Design review of the part built by this model. Coordinates are the model's own, in mm. Face numbers are marked on the shaded views. Give positions to 0.01 mm unless a question says otherwise; leave off trailing zeros. Order: outer loops, then holes, each group sorted by start corner. A loop starts at its lowest first (then second) coordinate and runs counter-clockwise, first axis right, second up. Notation, with made-up numbers: (18, -31) -> (59, -31) arc R11 cw to (59, -16) -> close; hole circle Ø10 at (40.5, -26.5). An arc over 180 degrees is marked (long way). Return JSON: item names as keys, results as strings.
```python
from build123d import *

# Parameters (mm, degrees)
SKETCH1_R           = 35.814
SKETCH1_R_2         = 2.032
BOSS_EXTRUDE1_DEPTH = 50.292
SKETCH2_R           = 13.716
CUT_EXTRUDE1_DEPTH  = 31.75
FILLET1_R           = 2.032


with BuildPart() as part:
    # Sketch1 → Boss-Extrude1 (new body)
    with BuildSketch(Plane(origin=(0, 0, 0), x_dir=(1, 0, 0), z_dir=(0, 1, 0))):
        with Locations(Location((0, 0, 0), (0, 0, 270))):
            Circle(SKETCH1_R)
        with Locations(Location((-20.308177359, -15.255750796, 0), (0, 0, 270))):
            Circle(SKETCH1_R_2, mode=Mode.SUBTRACT)
        with Locations(Location((-3.057779064, 25.215272896, 0), (0, 0, 270))):
            Circle(SKETCH1_R_2, mode=Mode.SUBTRACT)
        with Locations(Location((23.365956423, -9.959522099, 0), (0, 0, 270))):
            Circle(SKETCH1_R_2, mode=Mode.SUBTRACT)
    extrude(amount=BOSS_EXTRUDE1_DEPTH)

    # Sketch2 → Cut-Extrude1 (cut)
    with BuildSketch(Plane(origin=(0, 50.292, 0), x_dir=(1, 0, 0), z_dir=(0, 1, 0))):
        with Locations(Location((0, 0, 0), (0, 0, 270))):
            Circle(SKETCH2_R)
    extrude(amount=-CUT_EXTRUDE1_DEPTH, mode=Mode.SUBTRACT)

    # Fillet1
    fillet1_edges = [part.edges().sort_by_distance(p)[0] for p in [
        (0, 50.292, -35.814),
    ]]
    fillet(fillet1_edges, radius=FILLET1_R)


solid = part.part
```
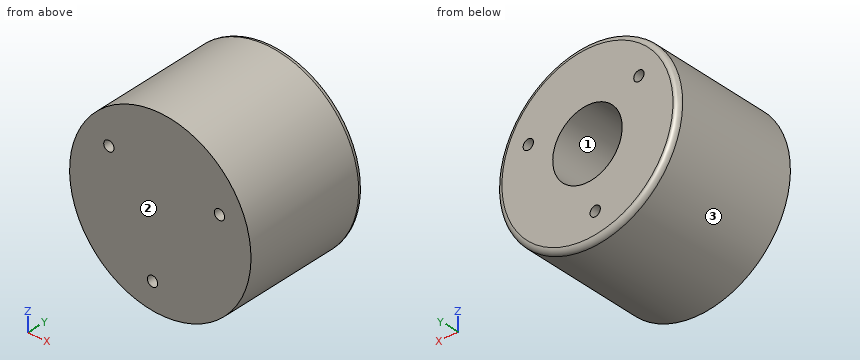
Item 1: Add section A-A (z = 0). Give the boundary of the cut face in (x, y).
Result set:
{"outline": "(-35.81, 0) -> (35.81, 0) -> (35.81, 48.26) arc R2.03 ccw to (33.78, 50.29) -> (13.72, 50.29) -> (13.72, 18.54) -> (-13.72, 18.54) -> (-13.72, 50.29) -> (-33.78, 50.29) arc R2.03 ccw to (-35.81, 48.26) -> close"}
Item 2: For pin 1 (8 mm diameter, centred on x = -4.5, y = 7.5, fed in from +Z); pin 2 (1 mm diameter, centred on x = -14.5, y = 14, fed in from -Z); pin 3 (5 mm diameter, centred on x = 23, y = 18.5, fed in from +Z); pin 4 (3.5 mm diameter, centred on x = -3.06, z = -25.22, fed in from +Y), all flat-tipped, find the tip position at first contact; note any pin that passes through.
Result set:
{"pin 1": "stops at z = 35.81", "pin 2": "stops at z = -32.96", "pin 3": "stops at z = 29.37", "pin 4": "passes through"}
Item 3: Add section B-B (x = 0). Give the boundary of the cut face in (y, z), plus the area to 3 significant figures.
Result set:
{"outline": "(0, -35.81) -> (48.26, -35.81) arc R2.03 ccw to (50.29, -33.78) -> (50.29, -13.72) -> (18.54, -13.72) -> (18.54, 13.72) -> (50.29, 13.72) -> (50.29, 33.78) arc R2.03 ccw to (48.26, 35.81) -> (0, 35.81) -> close", "area": "2,730 mm^2"}
Item 4: Mouldability with a two-part tool opening along X and no side actions: class the marked faces 1, 2 and 3 as released by +X, released by -X, zero draft, split by the parting line, or undercut.
Result set:
{"face 1": "undercut", "face 2": "zero draft", "face 3": "split by the parting line"}
Item 5: Add section C-C (y = 45). Give the boundary of the cut face in (x, z), plus the area to 3 significant figures.
Result set:
{"outline": "circle Ø71.63 at (0, 0); hole circle Ø4.06 at (-20.31, 15.26); hole circle Ø27.43 at (0, 0); hole circle Ø4.06 at (-3.06, -25.22); hole circle Ø4.06 at (23.37, 9.96)", "area": "3,400 mm^2"}
Item 6: Wall thickness on L1, parallel to X at y = 27, z = 0; L2, parallel to X at y = 26, z = 11.5; L3, parallel to Z at x = 10, y = 33: over which ranges is each line inside the solid? List them lowest first. Write a range as [from, to].
Result set:
{"L1": "x = [-35.81, -13.72], [13.72, 35.81]", "L2": "x = [-33.92, -7.48], [7.48, 22.04], [24.69, 33.92]", "L3": "z = [-34.39, -9.39], [9.39, 34.39]"}
Item 7: Add section D-D (y = 17.5). Give the boundary of the cut face in (x, z).
Result set:
{"outline": "circle Ø71.63 at (0, 0); hole circle Ø4.06 at (-20.31, 15.26); hole circle Ø4.06 at (-3.06, -25.22); hole circle Ø4.06 at (23.37, 9.96)"}
